Job drawing, mm, ordinate dimensions from the low corner. One solid piece. A direction names the side the tool comes from. Give positions to 0.01 mm unless a question says otherwise; leave off trailing zeros. Write each loop counter-clockwise with the first axis right and the second up, starting at its lowest first coordinate (ties: lowest second). Pieces come first, ordered by that corner, then holes. Notation, with made-up numbers: M 29.25,-4.5 L 40.25,-4.5 A21 cw 40.25,29.5 Z; hole C 87.25,50.5 d3. An arc over 180 degrees is marked long. Answer as CSV lines item,"result". Start each with the question number.
1) Tool access for the marked faces 5, 6 and 7: list every direction of +Z, -Z, +X, -X, +Y, -Y with a clear straight run to the whole face (end or side of a thin tool).
2) Wall check: line 1 along X through (y, z) = (10, 6.5); line 2 along Y through (x, z) = (23.8, 5.25); line 3 along Z through (x, y) = (37, 2.5). Give the ranges that are in metal, low to high. Write a range as from..to.
3) Pin check, flat tips, straight feed: pin 1 Ø5.5 at (y, z) = (6.5, 4) entering from -X; pin 2 Ø3 at (y, z) = (15, 18) entering from -X; pin 3 Ø3 at (x, y) = (33.5, 5) entering from +Z. Stop position of each tip, or through.
4) Mould opens along X. For the marked faces 1, 2, 3 and 4 say: pulls with the +X half, pulls with the -X half, needs draft (parallel to the pull), parting line crosses it, or undercut.
5) Slice it at B-B, the plane z = 5.5. Give the cut face in (x, y).
6) Slice it at C-C, the plane x = 23.8. Give the cut face in (y, z), plus the area to 3 significant figures.
7) Slice it at D-D, the plane z = 7.5. Give the cut face in (x, y), plus the area to 3 significant figures.
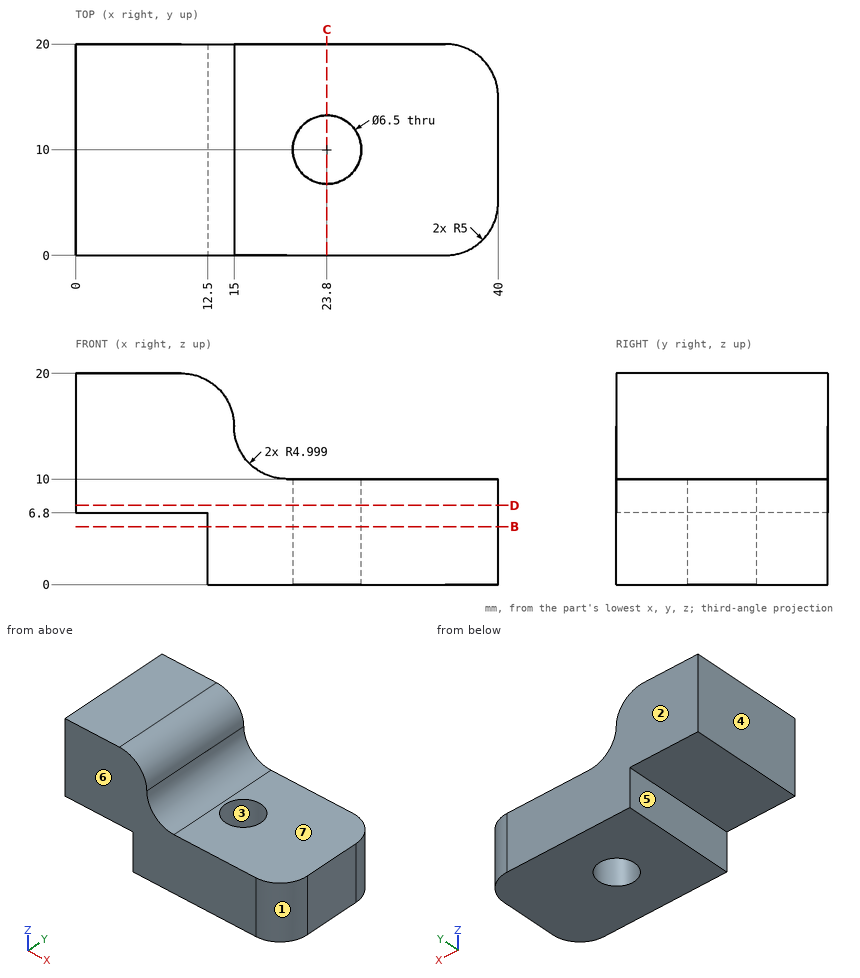
Found:
1,face 5,"-Z, -X, +Y, -Y"
1,face 6,"+Z, -Z, +X, -X, -Y"
1,face 7,"+Z, +X, +Y, -Y"
2,line 1,"12.5..20.55, 27.05..40"
2,line 2,"0..6.75, 13.25..20"
2,line 3,"0..10"
3,pin 1,"x = 12.5"
3,pin 2,"x = 0"
3,pin 3,"z = 10"
4,face 1,"pulls with the +X half"
4,face 2,"needs draft"
4,face 3,"undercut"
4,face 4,"pulls with the -X half"
5,outline,"M 12.5,0 L 35,0 A5 ccw 40,5 L 40,15 A5 ccw 35,20 L 12.5,20 Z; hole C 23.8,10 d6.5"
6,outline,"M 0,0 L 6.75,0 L 6.75,10 L 0,10 Z; M 13.25,0 L 20,0 L 20,10 L 13.25,10 Z"
6,area,"135 mm²"
7,outline,"M 0,0 L 35,0 A5 ccw 40,5 L 40,15 A5 ccw 35,20 L 0,20 Z; hole C 23.8,10 d6.5"
7,area,"756 mm²"
